```python
from build123d import *

# Parameters (mm, degrees)
SKETCH1_R                       = 4.7625
EXTRUDE1_DEPTH                  = 19.05
SKETCH2_R                       = 3.0607
CUT_EXTRUDE1_DEPTH              = 10.414
SKETCH3_R                       = 3.4925
CUT_EXTRUDE2_DEPTH              = 0.635
CUT_EXTRUDE5_DEPTH              = 6.35
F_9_64_0_14063_DIAMETER_HOLE1_D = 3.57124
SKETCH7_W                       = 9.525
SKETCH7_H                       = 1.5875
CUT_EXTRUDE4_DEPTH              = 0.635


with BuildPart() as part:
    # Sketch1 → Extrude1 (new body)
    with BuildSketch(Plane(origin=(0, 0, 0), x_dir=(1, 0, 0), z_dir=(0, 1, 0))):
        with Locations(Location((0, 0, 0), (0, 0, 270))):  # turned: the seam where the file's is
            Circle(SKETCH1_R)
    extrude(amount=EXTRUDE1_DEPTH)

    # Sketch2 → Cut-Extrude1 (cut)
    with BuildSketch(Plane(origin=(0, 19.05, 0), x_dir=(1, 0, 0), z_dir=(0, 1, 0))):
        with Locations(Location((0, 0, 0), (0, 0, 270))):  # turned: the seam where the file's is
            Circle(SKETCH2_R)
    extrude(amount=-CUT_EXTRUDE1_DEPTH, mode=Mode.SUBTRACT)

    # Sketch3 → Cut-Extrude2 (cut)
    with BuildSketch(Plane.XZ):
        with Locations(Location((0, 0, 0), (0, 0, 270))):  # turned: the seam where the file's is
            Circle(SKETCH3_R)
    extrude(amount=-CUT_EXTRUDE2_DEPTH, mode=Mode.SUBTRACT)

    # Sketch8 → Cut-Extrude5 (cut)
    with BuildSketch(Plane(origin=(0, 19.05, 0), x_dir=(1, 0, 0), z_dir=(0, 1, 0))):
        with BuildLine():
            Line((-1.825754756, 3.1877), (-3.673506558, -0.0127))
            ThreePointArc((-3.673506558, -0.0127), (-3.673506558, -2.1209), (-1.847751802, -3.175))
            Line((-1.847751802, -3.175), (1.847751802, -3.175))
            ThreePointArc((1.847751802, -3.175), (3.673506558, -2.1209), (3.673506558, -0.0127))
            Line((3.673506558, -0.0127), (1.825754756, 3.1877))
            ThreePointArc((1.825754756, 3.1877), (0, 4.2418), (-1.825754756, 3.1877))
        make_face()
    extrude(amount=-CUT_EXTRUDE5_DEPTH, mode=Mode.SUBTRACT)

    # 9/64 (0.14063) Diameter Hole1 (through all)
    with Locations(Plane(origin=(0, 0.635, 0), x_dir=(0, 0, -1), z_dir=(0, -1, 0))):
        with Locations((0, 0)):
            Hole(F_9_64_0_14063_DIAMETER_HOLE1_D / 2)

    # Sketch7 → Cut-Extrude4 (cut)
    with BuildSketch(Plane.XZ):
        Rectangle(SKETCH7_W, SKETCH7_H)
    extrude(amount=-CUT_EXTRUDE4_DEPTH, mode=Mode.SUBTRACT)


solid = part.part
```
Design review of the part built by this model. Coordinates are the model's own, in mm. A direction names the side the tool comes from. Coordinates: 2 decimals unless noted, no trailing zeros. Loops run counter-clockwise (first coordinate to the right, second up) from the corner with the lowest first, then second, coordinate; pieces in that order, holes last. Notation, with made-up numbers: (13.5, 52) - (17.5, 52) arc R18 ccw to (17.5, 76) - close; hole circle Ø10 at (-23.5, 21). An arc over 180 degrees is marked (long way). Use CSV: the item, a comma, the result in double quotes. Start each with the question number.
1) Consider section B-B on y = 18. Write out the cut boundary in (x, z) (1 decimal), then the cut area to 3 significant figures.
2) Tool access review of faces 1 (the flat face through (3, 12.7, 2)), 2 (the flat face through (-2.4, 19.05, -2.5)), 3 (the cylindrical face through (0.07, 0.31, 3.49)): name each direction out of +Z, -Z, +X, -X, +Y, -Y from which nothing blocks a thin tool from reaching the whole face with its end or side.
3) The part is to be moulded in two halves that separate along Z. For faces 4 (the cylindrical face through (-0.07, 0.31, -3.49)), 5 (the cylindrical face through (-2.9, 9.39, -3.78)), 6 (the flat face through (0, 0, -4)), say which applies: +Z half, -Z half, draft (parallel to the pull), parting line (faces both ways), or undercut.
4) Consider section D-D on z = -2.25. Write out the cut boundary in (x, y) (3 decimals).
5) Wall thickness on L1, parallel to X at y = 6.25, z = 0; L2, parallel to X at y = 9.9, z = 0; L3, parallel to Y at x = 0.5, z = -3.75: over which ranges is each line inside the solid? List them lowest first. Write a range as from..to.
6) For pin 1 Ø4.5 at (x, z) = (0, 0) entering from +Y; pin 2 Ø2 at (x, y) = (1.5, 4.5) entering from -Z; pin 3 Ø1 at (y, z) = (17, 2.5) entering from +X, all flat-tipped, find the tip position at first contact; note any pin that passes through.
Geometry says:
1,outline,"circle Ø9.5 at (0, 0); hole (-3.7, 0) - (-1.8, -3.2) arc R2.1 ccw to (1.8, -3.2) - (3.7, 0) arc R2.1 ccw to (1.8, 3.2) - (-1.8, 3.2) arc R2.1 ccw to start"
1,area,"28.0 mm^2"
2,face 1,"+Y"
2,face 2,"+Z, -Z, +X, -X, +Y"
2,face 3,"-Y"
3,face 4,"undercut"
3,face 5,"parting line"
3,face 6,"draft"
4,outline,"(-4.197, 0) - (-2.671, 0) - (-2.671, 0.635) - (2.671, 0.635) - (2.671, 0) - (4.197, 0) - (4.197, 19.05) - (2.367, 19.05) - (2.367, 12.7) - (2.075, 12.7) - (2.075, 8.636) - (-2.075, 8.636) - (-2.075, 12.7) - (-2.367, 12.7) - (-2.367, 19.05) - (-4.197, 19.05) - close"
5,L1,"-4.76..-1.79, 1.79..4.76"
5,L2,"-4.76..-3.06, 3.06..4.76"
5,L3,"0..12.7"
6,pin 1,"y = 8.64"
6,pin 2,"z = -4.74"
6,pin 3,"x = 4.32"
